Here's how the part is built. I have some questions about the finished solid (model axes, mm). A direction names the side the tool comes from. Coordinates: 2 decimals unless noted, no trailing zeros. Loops run counter-clockwise (first coordinate to the right, second up) from the corner with the lowest first, then second, coordinate; pieces in that order, holes last. Notation, with made-up numbers: M 14.25,60 L 67.25,60 A12 ccw 67.25,78 Z; hole C -9.75,15 d1. An arc over 180 degrees is marked long. Use CSV: the item, a comma, the result in double quotes. Start each with the question number.
Q1. If we mould it in two halves opening along Z, with no side actions, what happens to faces 5 (the flat face through (1, 26, -20)), 6 (the flat face through (1.257, 12.533, -7.444)), 7 (the flat face through (-39, 21, -8))? For each: +Z half, -Z half, draft (parallel to the pull), parting line (faces both ways), or undercut.
Q2. If we section it at B-B (z = -16.5): Please give me the cut outline in (x, y), and give its area (3 significant figures).
Q3. Please list where these lines run through material, in increasing order: probe 1 along Y at (x, z) = (35, -6.75); probe 2 along Y at (x, z) = (22, -17.75); probe 3 along Z at (x, y) = (31, -3.5). Write a range as [from, to].
Q4. If we section it at C-C (y = 30): Please give me the cut outline in (x, z).
Q5. Which directions (+Z, -Z, +X, -X, +Y, -Y) give clear straight access to the entire face, cutting with the end or side of a thin tool? Please do faces 1 (the cylindrical face through (-3.48, 10.4, -14.1)), 2 (the flat face through (48, -4.5, -7)), 3 (the flat face through (-18.08, -4.17, -7.4)), 4 (the flat face through (17.894, 7.066, -0.986)).
Q6. If we section it at D-D (z = -7.5): State how many separate pieces and enclosed holes the cut face has, and give its area (3 significant figures).
Q7. For pin 1 Ø9 at (x, z) = (-42.5, -5.5) entering from -Y; pin 2 Ø12 at (x, z) = (0.5, -13) entering from +Y; pin 3 Ø4.5 at (x, y) = (-17, 38.5) entering from -Z; pin 4 Ø3 at (x, y) = (-27.4, 35.5) entering from -Z, each with a flat end and sliding along its axis, tell me the tip position at first contact or that it passes through.
from build123d import *

# Parameters (mm, degrees)
BOSS_EXTRUDE1_DEPTH = 15
CUT_EXTRUDE1_START  = -13
CUT_EXTRUDE1_DEPTH  = 13
BOSS_EXTRUDE2_DEPTH = 13
SKETCH5_R           = 4
CUT_EXTRUDE2_DEPTH  = 18
SKETCH6_W           = 78
SKETCH6_H           = 5
BOSS_EXTRUDE3_DEPTH = 15
SKETCH7_W           = 78
SKETCH7_H           = 5
BOSS_EXTRUDE4_DEPTH = 5
CUT_EXTRUDE3_REACH  = 69.479
SKETCH8_R           = 1.6
CUT_EXTRUDE4_REACH  = 67.18
SKETCH9_R           = 1.6
CHAMFER1_SIZE       = 5
FILLET1_R           = 3
FILLET2_R           = 3
SKETCH10_R          = 1.6
CUT_EXTRUDE5_DEPTH  = 72.66390448


with BuildPart() as part:
    # Sketch2 → Boss-Extrude1 (new body)
    with BuildSketch(Plane.XY):
        with BuildLine():
            Line((-39, 28), (39, 28))
            Line((39, 28), (39, 8.062257748))
            ThreePointArc((39, 8.062257748), (41.160225429, 6.561373535), (42.794228634, 4.5))
            Line((42.794228634, 4.5), (49.794228634, 4.5))
            Line((49.794228634, 4.5), (49.794228634, 1.5))
            Line((49.794228634, 1.5), (38.708099244, 1.5))
            ThreePointArc((38.708099244, 1.5), (31, 0), (38.708099244, -1.5))
            Line((38.708099244, -1.5), (49.794228634, -1.5))
            Line((49.794228634, -1.5), (49.794228634, -4.5))
            Line((49.794228634, -4.5), (42.794228634, -4.5))
            ThreePointArc((42.794228634, -4.5), (32.868581203, -8.743972433), (26.009276503, -0.408522957))
            Line((26.009276503, -0.408522957), (-9.429697367, -8.278133847))
            Line((-9.429697367, -8.278133847), (-26.009276503, -0.408522957))
            ThreePointArc((-26.009276503, -0.408522957), (-32.868581203, -8.743972433), (-42.794228634, -4.5))
            Line((-42.794228634, -4.5), (-49.794228634, -4.5))
            Line((-49.794228634, -4.5), (-49.794228634, -1.5))
            Line((-49.794228634, -1.5), (-38.708099244, -1.5))
            ThreePointArc((-38.708099244, -1.5), (-31, 0), (-38.708099244, 1.5))
            Line((-38.708099244, 1.5), (-49.794228634, 1.5))
            Line((-49.794228634, 1.5), (-49.794228634, 4.5))
            Line((-49.794228634, 4.5), (-42.794228634, 4.5))
            ThreePointArc((-42.794228634, 4.5), (-41.160225429, 6.561373535), (-39, 8.062257748))
            Line((-39, 8.062257748), (-39, 28))
        make_face()
        Polygon((-10.513599328, -3.397031867), (-12.247842467, 4.4127313), (17.038769412, 10.916143071), (18.773012551, 3.106379903), align=None, mode=Mode.SUBTRACT)
    extrude(amount=-BOSS_EXTRUDE1_DEPTH)

    # Sketch3 → Cut-Extrude1 (cut)
    with BuildSketch(Plane(origin=(0, 0, -15), x_dir=(-1, 0, 0), z_dir=(0, 0, -1)).offset(CUT_EXTRUDE1_START)):
        with BuildLine():
            Line((-34, 8.94427191), (-34, 23))
            Line((-34, 23), (34, 23))
            Line((34, 23), (34, 8.94427191))
            ThreePointArc((34, 8.94427191), (30.031333309, 7.504155603), (27.156034009, 4.4127313))
            Line((27.156034009, 4.4127313), (12.247842467, 4.4127313))
            Line((12.247842467, 4.4127313), (10.513599328, -3.397031867))
            Line((10.513599328, -3.397031867), (-27.55471368, 5.056452473))
            ThreePointArc((-27.55471368, 5.056452473), (-30.351398032, 7.706523194), (-34, 8.94427191))
        make_face()
    extrude(amount=CUT_EXTRUDE1_DEPTH, mode=Mode.SUBTRACT)

    # Sketch4 → Boss-Extrude2 (add)
    with BuildSketch(Plane(origin=(0, 0, -2), x_dir=(-1, 0, 0), z_dir=(0, 0, -1))):
        Polygon((-8.252785849, 8.96511954), (-6.51854271, 16.774882707), (5.196102042, 14.173517999), (3.461858903, 6.363754831), align=None)
    extrude(amount=BOSS_EXTRUDE2_DEPTH)

    # Sketch5 → Cut-Extrude2 (cut)
    with BuildSketch(Plane(origin=(1.308726989, -5.893549531, 0), x_dir=(0.9762203959642156, 0.21678039234089003, 0), z_dir=(0.21678039234089003, -0.9762203959642156, 0))):
        with Locations((4, -7.5)):
            Circle(SKETCH5_R)
    extrude(amount=-CUT_EXTRUDE2_DEPTH, mode=Mode.SUBTRACT)

    # Sketch6 → Boss-Extrude3 (add)
    with BuildSketch(Plane(origin=(0, 28, 0), x_dir=(1, 0, 0), z_dir=(0, 1, 0))):
        with Locations((0, 2.5)):
            Rectangle(SKETCH6_W, SKETCH6_H)
    extrude(amount=BOSS_EXTRUDE3_DEPTH)

    # Sketch7 → Boss-Extrude4 (add)
    with BuildSketch(Plane(origin=(0, 0, -15), x_dir=(-1, 0, 0), z_dir=(0, 0, -1))):
        with Locations((0, 25.5)):
            Rectangle(SKETCH7_W, SKETCH7_H)
    extrude(amount=BOSS_EXTRUDE4_DEPTH)

    # Sketch8 → Cut-Extrude3 (cut, up to next)
    with BuildSketch(Plane(origin=(0, 0, -5), x_dir=(-1, 0, 0), z_dir=(0, 0, -1)), mode=Mode.PRIVATE) as cut_extrude3_sk1:
        with Locations((27.4, 35.5)):
            Circle(SKETCH8_R)
    cut_extrude3_tool1 = extrude(cut_extrude3_sk1.sketch, amount=-CUT_EXTRUDE3_REACH, mode=Mode.PRIVATE) & part.part
    # Sketch8 → Cut-Extrude3 (cut, up to next)
    with BuildSketch(Plane(origin=(0, 0, -5), x_dir=(-1, 0, 0), z_dir=(0, 0, -1)), mode=Mode.PRIVATE) as cut_extrude3_sk2:
        with Locations((-27.4, 35.5)):
            Circle(SKETCH8_R)
    cut_extrude3_tool2 = extrude(cut_extrude3_sk2.sketch, amount=-CUT_EXTRUDE3_REACH, mode=Mode.PRIVATE) & part.part
    add(cut_extrude3_tool1.solids().sort_by_distance((-27.4, 35.5, -5))[0], mode=Mode.SUBTRACT)
    add(cut_extrude3_tool2.solids().sort_by_distance((27.4, 35.5, -5))[0], mode=Mode.SUBTRACT)

    # Sketch9 → Cut-Extrude4 (cut, up to next)
    with BuildSketch(Plane(origin=(0, 28, 0), x_dir=(1, 0, 0), z_dir=(0, 1, 0)), mode=Mode.PRIVATE) as cut_extrude4_sk1:
        with Locations(Location((-27.4, 12.5, 0), (0, 0, 270))):
            Circle(SKETCH9_R)
    cut_extrude4_tool1 = extrude(cut_extrude4_sk1.sketch, amount=-CUT_EXTRUDE4_REACH, mode=Mode.PRIVATE) & part.part
    # Sketch9 → Cut-Extrude4 (cut, up to next)
    with BuildSketch(Plane(origin=(0, 28, 0), x_dir=(1, 0, 0), z_dir=(0, 1, 0)), mode=Mode.PRIVATE) as cut_extrude4_sk2:
        with Locations(Location((27.4, 12.5, 0), (0, 0, 270))):
            Circle(SKETCH9_R)
    cut_extrude4_tool2 = extrude(cut_extrude4_sk2.sketch, amount=-CUT_EXTRUDE4_REACH, mode=Mode.PRIVATE) & part.part
    add(cut_extrude4_tool1.solids().sort_by_distance((-27.4, 28, -12.5))[0], mode=Mode.SUBTRACT)
    add(cut_extrude4_tool2.solids().sort_by_distance((27.4, 28, -12.5))[0], mode=Mode.SUBTRACT)

    # Chamfer1
    chamfer1_edges = [part.edges().sort_by_distance(p)[0] for p in [
        (36.5, 23, -15),
        (-36.5, 23, -15),
    ]]
    chamfer(chamfer1_edges, length=CHAMFER1_SIZE - 0.0001)  # a hair under: the kernel refuses the full size

    # Fillet1
    fillet1_edges = [part.edges().sort_by_distance(p)[0] for p in [
        (-4.328980472, 10.268636415, -15),
        (0.661220334, 15.474200353, -15),
        (7.385664279, 12.870001123, -15),
    ]]
    fillet(fillet1_edges, radius=FILLET1_R)

    # Fillet2
    fillet2_edges = [part.edges().sort_by_distance(p)[0] for p in [
        (-9.429697367, -8.278133847, -7.5),
    ]]
    fillet(fillet2_edges, radius=FILLET2_R)

    # Sketch10 → Cut-Extrude5 (cut, through all)
    with BuildSketch(Plane.XZ.offset(4.5)):
        with Locations(Location((46.294228634, -7.5, 0), (0, 0, 270))):
            Circle(SKETCH10_R)
        with Locations((-46.294228634, -7.5)):
            Circle(SKETCH10_R)
    extrude(amount=-CUT_EXTRUDE5_DEPTH, mode=Mode.SUBTRACT)


solid = part.part
Results below:
1,face 5,"-Z half"
1,face 6,"undercut"
1,face 7,"draft"
2,outline,"M -39,19.5 L -34,19.5 L -34,23 L 34,23 L 34,19.5 L 39,19.5 L 39,28 L -39,28 Z"
2,area,"425 mm^2"
3,probe 1,"[-9, -4], [4, 28]"
3,probe 2,"[23, 28]"
3,probe 3,"[-15, 0]"
4,outline,"M -39,-5 L 39,-5 L 39,0 L -39,0 Z"
5,face 1,"-Z"
5,face 2,"+Z, -Z, +X, -Y"
5,face 3,"+Z, -Z, -Y"
5,face 4,"+Z, -Z"
6,separate pieces,"6"
6,enclosed holes,"0"
6,area,"1,280 mm^2"
7,pin 1,"y = -8.49"
7,pin 2,"y = 28"
7,pin 3,"z = -5"
7,pin 4,"through"
